Input: dimensioned drawing with shaded views. Units: mm. Origin: part minimum x, y, z. Round coordinates to 2 decimals unless told otherwise and drop trailing zeros. Order: outer loops, then holes, each group sorted by start corner. A loop starts at its lowest first (then second) coordinate and runs counter-clockwise, first axis right, second up.
Item 1: Line query: L1, parallel to X at y = 6.5, z = 6; L2, parallel to Z at x = 7.5, y = 2.75; L3, parallel to X at y = 1.4, z = 29. Output: solid intervals per line, ascending.
Item 2: Cut plane D-D on y = 3. Output: boundary loops of the cut face in (x, z), then the cut area to 3 significant figures.
Item 3: Cut plane C-C on x = 8. Output: boundary loops of the cut face in (y, z), then the cut area to 3 significant figures.
Item 4: Cut plane B-B on y = 6. Output: boundary loops of the cut face in (x, z), then the cut area to 3 significant figures.
Item 5: Cut plane A-A on z = 17.5. Output: boundary loops of the cut face in (x, y), then the cut area to 3 significant figures.
Item 6: Mould query, pull axis X, two halves, no side actions, for the marked faces 1, 2, 3 and 4. Classes: released by +X, released by -X, zero draft, split by the parting line, or undercut.
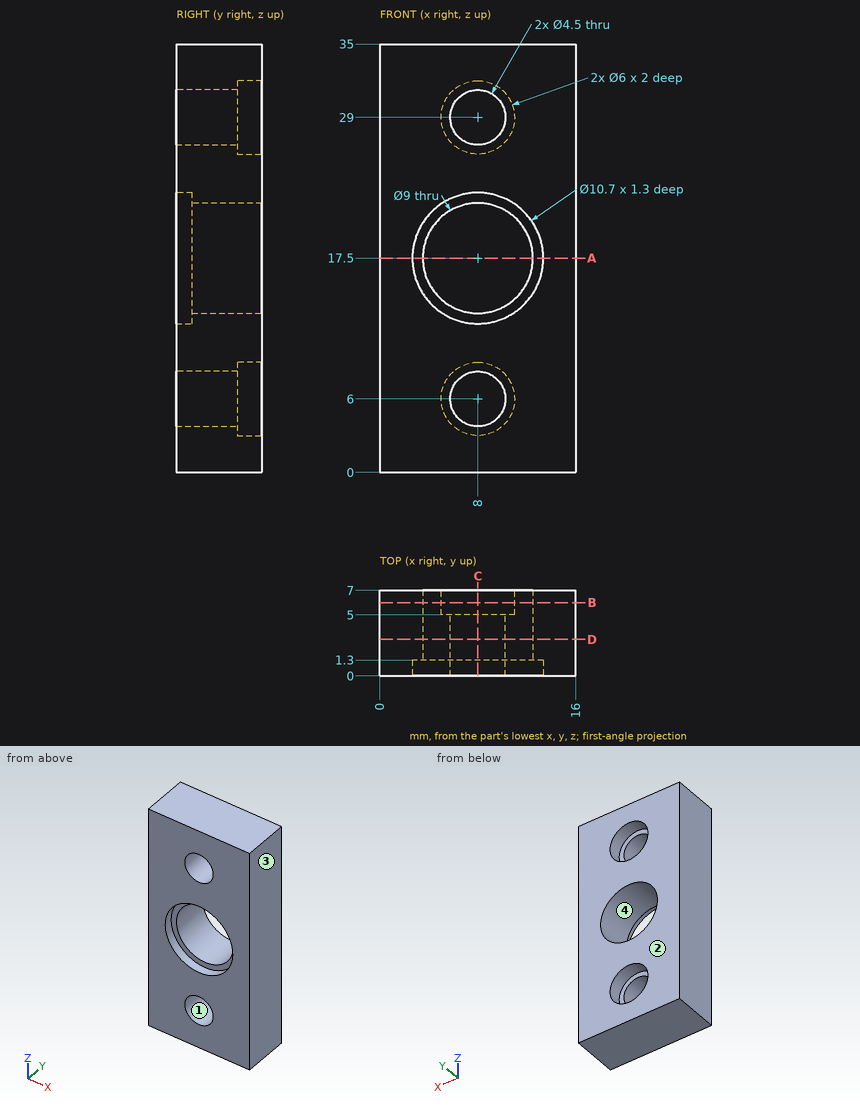
From the geometry:
1. L1: x = 0 to 5, 11 to 16
1. L2: z = 0 to 3.81, 8.19 to 13.03, 21.97 to 26.81, 31.19 to 35
1. L3: x = 0 to 5.75, 10.25 to 16
2. outline: (0, 0) - (16, 0) - (16, 35) - (0, 35) - close; hole circle Ø9 at (8, 17.5); hole circle Ø4.5 at (8, 6); hole circle Ø4.5 at (8, 29)
2. area: 465 mm2
3. outline: (0, 0) - (7, 0) - (7, 3) - (5, 3) - (5, 3.75) - (0, 3.75) - close; (0, 8.25) - (5, 8.25) - (5, 9) - (7, 9) - (7, 13) - (1.3, 13) - (1.3, 12.15) - (0, 12.15) - close; (0, 22.85) - (1.3, 22.85) - (1.3, 22) - (7, 22) - (7, 26) - (5, 26) - (5, 26.75) - (0, 26.75) - close; (0, 31.25) - (5, 31.25) - (5, 32) - (7, 32) - (7, 35) - (0, 35) - close
3. area: 111 mm2
4. outline: (0, 0) - (16, 0) - (16, 35) - (0, 35) - close; hole circle Ø9 at (8, 17.5); hole circle Ø6 at (8, 6); hole circle Ø6 at (8, 29)
4. area: 440 mm2
5. outline: (0, 0) - (2.65, 0) - (2.65, 1.3) - (3.5, 1.3) - (3.5, 7) - (0, 7) - close; (12.5, 1.3) - (13.35, 1.3) - (13.35, 0) - (16, 0) - (16, 7) - (12.5, 7) - close
5. area: 46.8 mm2
6. face 1: undercut
6. face 2: zero draft
6. face 3: released by +X
6. face 4: undercut
